```python
from build123d import *

# Parameters (mm, degrees)
BOSS_EXTRUDE1_DEPTH     = 18
CUT_EXTRUDE1_DEPTH      = 44.04814257
CUT_EXTRUDE1_DEPTH_BACK = 44.04814257
SKETCH5_R               = 1.5
CUT_EXTRUDE2_DEPTH      = 44.048142727
CUT_EXTRUDE3_START      = -18
CUT_EXTRUDE3_DEPTH      = 18
FILLET1_R               = 2
CUT_EXTRUDE5_REACH      = 44.569


# Read off the part's stored shape, not the designer's step: Cut-Extrude3
with BuildPart() as part:
    # Sketch2 → Boss-Extrude1 (new body)
    with BuildSketch(Plane(origin=(0, 0, 0), x_dir=(1, 0, 0), z_dir=(0, 1, 0))):
        with BuildLine():
            Line((5.149404736, 36.639918543), (4.036019928, 28.717773994))
            Line((4.036019928, 28.717773994), (-9.918584156, 27.251086003))
            Line((-9.918584156, 27.251086003), (-12.654745303, 34.768626969))
            ThreePointArc((-12.654745303, 34.768626969), (-3.867553141, 36.797310129), (5.149404736, 36.639918543))
        make_face()
    extrude(amount=BOSS_EXTRUDE1_DEPTH)

    # Sketch3 → Cut-Extrude1 (cut, two sides: drawn at the far end of the back side and taken through both)
    with BuildSketch(Plane(origin=(0, 0, 0), x_dir=(0, 0, -1), z_dir=(1, 0, 0)).offset(-CUT_EXTRUDE1_DEPTH_BACK)):
        with BuildLine():
            Line((38, 13.1), (41.639918543, 13.1))
            Line((41.639918543, 13.1), (41.639918543, 4.9))
            Line((41.639918543, 4.9), (38, 4.9))
            ThreePointArc((38, 4.9), (33.9, 9), (38, 13.1))
        make_face()
    extrude(amount=CUT_EXTRUDE1_DEPTH + CUT_EXTRUDE1_DEPTH_BACK, mode=Mode.SUBTRACT)

    # Sketch5 → Cut-Extrude2 (cut, through all)
    with BuildSketch(Plane.XY):
        with Locations(Location((0, 3.1, 0), (0, 0, 90))):
            Circle(SKETCH5_R)
        with Locations(Location((0, 14.9, 0), (0, 0, 90))):
            Circle(SKETCH5_R)
    extrude(amount=-CUT_EXTRUDE2_DEPTH, mode=Mode.SUBTRACT)

    # Cut-Extrude3 outline → Cut-Extrude3 (cut)
    with BuildSketch(Plane(origin=(0, 18, 0), x_dir=(1, 0, 0), z_dir=(0, 1, 0)).offset(CUT_EXTRUDE3_START)):
        with BuildLine():
            ThreePointArc((-12.483737701, 34.29877976), (-3.815290216, 36.300049044), (5.079818185, 36.144784509))
            Line((5.079818185, 36.144784509), (5.149404736, 36.639918543))
            ThreePointArc((5.149404736, 36.639918543), (-3.867553141, 36.797310129), (-12.654745303, 34.768626969))
            Line((-12.654745303, 34.768626969), (-12.483737701, 34.29877976))
        make_face()
    extrude(amount=CUT_EXTRUDE3_DEPTH, mode=Mode.SUBTRACT)

    # Fillet1
    fillet1_edges = [part.edges().sort_by_distance(p)[0] for p in [
        (4.557919056, 18, -32.431279251),
        (4.557919056, 0, -32.431279251),
        (-11.201159694, 0, -30.774933331),
        (-11.201159694, 18, -30.774933331),
    ]]
    fillet(fillet1_edges, radius=FILLET1_R)

    # Cut-Extrude5: up to this plane
    cut_extrude5_end = Plane(origin=(-10.179905315, 18, -29.737390741), z_dir=(-0.10452846326765396, 0, -0.9945218953682733))
    # Sketch7 → Cut-Extrude5 (cut, up to the surface)
    with BuildSketch(Plane.XY, mode=Mode.PRIVATE) as cut_extrude5_sk1:
        Polygon((3.233161507, 14.9), (1.616580754, 17.7), (-1.616580754, 17.7), (-3.233161507, 14.9), (-1.616580754, 12.1), (1.616580754, 12.1), align=None)
    cut_extrude5_tool1 = split(extrude(cut_extrude5_sk1.sketch, amount=-CUT_EXTRUDE5_REACH, mode=Mode.PRIVATE), bisect_by=cut_extrude5_end, keep=Keep.BOTH, mode=Mode.PRIVATE)
    add(cut_extrude5_tool1.solids().sort_by_distance((0, 14.9, 0))[0], mode=Mode.SUBTRACT)
    # Sketch7 → Cut-Extrude5 (cut, up to the surface)
    with BuildSketch(Plane.XY, mode=Mode.PRIVATE) as cut_extrude5_sk2:
        Polygon((-3.233161507, 3.1), (-1.616580754, 0.3), (1.616580754, 0.3), (3.233161507, 3.1), (1.616580754, 5.9), (-1.616580754, 5.9), align=None)
    cut_extrude5_tool2 = split(extrude(cut_extrude5_sk2.sketch, amount=-CUT_EXTRUDE5_REACH, mode=Mode.PRIVATE), bisect_by=cut_extrude5_end, keep=Keep.BOTH, mode=Mode.PRIVATE)
    add(cut_extrude5_tool2.solids().sort_by_distance((0, 3.1, 0))[0], mode=Mode.SUBTRACT)


solid = part.part
```
The model under review builds one solid part; all positions refer to its coordinate system, in mm. A direction names the side the tool comes from. Round coordinates to 2 decimals unless told otherwise and drop trailing zeros. Loops run counter-clockwise (first coordinate to the right, second up) from the corner with the lowest first, then second, coordinate; pieces in that order, holes last. Notation, with made-up numbers: (-6, 6) - (24, 6) arc R4 ccw to (24, 10) - close; hole circle Ø4 at (24, 74.5). An arc over 180 degrees is marked (long way). Use a Markdown table: item, result. Add a question column.
Q1. Machinability: for faces 4 (the face through (0, 5.9, -30)), 5 (the face through (-4, 0, -32)), which of the approach directions +Z, -Z, +X, -X, +Y, -Y give a long, thin tool a straight path to every point of the face, cutting with its end or side? Answer none if there is none.
Q2. Add section A-A (x = 1.25). State the section outline as (y, z) points.
Q3. The part is to be moulded in two halves that separate along X. For faces 1 (the face through (-2.436, 13.52, -29.277)), 2 (the face through (-3.939, 15.135, -36.287)), 3 (the face through (-3.8, 8.9, -33.9)), say which applies: pulls with the +X half, pulls with the -X half, needs draft (parallel to the pull), parting line crosses it, or undercut.
Q4. Add section D-D (y = 14.25). State the section outline as (x, z) points, plus the area to 3 significant figures.
Q5. Add section C-C (x = -6.5). State the section outline as (y, z) points.
Q6. Insertion check: pin 1 Ø2 at (y, z) = (10, -30.5) entering from +X; pin 2 Ø2 at (x, y) = (1, 9.5) entering from -Z; pin 3 Ø2 at (y, z) = (3, -31) entering from -X; pin 4 Ø3 at (x, z) = (-10.5, -32) entering from -Y. Each pin has a flat end and moves straight along its axis. Give the tip position at first contact, or say it passes through.
Q7. For probe 1 along Y at (x, z) = (-2.5, -30.5); probe 2 along Y at (x, z) = (-2.25, -28.25); probe 3 along X at (y, z) = (3.1, -33.9), list the stretches that pass through material, from the lowest coordinate up.
Q8. Add section B-B (y = 2.5). State the section outline as (x, z) points.
Worked answers:
| question | item | result |
|---|---|---|
| 1 | face 4 | +Z |
| 1 | face 5 | +Z, -Z, +X, -X, -Y |
| 2 | outline | (0, -36.48) - (2.27, -36.48) - (2.27, -30.94) - (0.3, -30.94) - (0.3, -28.42) - (0, -28.42) - close; (3.93, -36.48) - (5.19, -36.48) arc R4.1 cw to (12.81, -36.48) - (14.07, -36.48) - (14.07, -30.94) - (12.1, -30.94) - (12.1, -28.42) - (5.9, -28.42) - (5.9, -30.94) - (3.93, -30.94) - close; (15.73, -36.48) - (18, -36.48) - (18, -28.42) - (17.7, -28.42) - (17.7, -30.94) - (15.73, -30.94) - close |
| 3 | face 1 | undercut |
| 3 | face 2 | parting line crosses it |
| 3 | face 3 | needs draft |
| 4 | outline | (-12.48, -34.3) arc R36.5 ccw to (-1.35, -36.47) - (-1.35, -30.67) - (-2.86, -30.51) - (-2.86, -27.99) - (-9.92, -27.25) - close; (1.35, -36.47) arc R36.5 ccw to (5.08, -36.14) - (4.04, -28.72) - (2.86, -28.59) - (2.86, -31.11) - (1.35, -30.95) - close |
| 4 | area | 98.4 mm² |
| 5 | outline | (0, -35.92) - (5.47, -35.92) arc R4.1 cw to (12.53, -35.92) - (18, -35.92) - (18, -27.61) - (0, -27.61) - close |
| 6 | pin 1 | x = 4.43 |
| 6 | pin 2 | z = -34.18 |
| 6 | pin 3 | x = -11.65 |
| 6 | pin 4 | y = 0 |
| 7 | probe 1 | 0 to 1.83, 4.37 to 13.63, 16.17 to 18 |
| 7 | probe 2 | 0 to 1.4, 4.8 to 13.2, 16.6 to 18 |
| 7 | probe 3 | -12.34 to -1.5, 1.5 to 4.76 |
| 8 | outline | (-12.48, -34.3) arc R36.5 ccw to (-1.37, -36.47) - (-1.37, -30.66) - (-2.89, -30.5) - (-2.89, -27.99) - (-9.92, -27.25) - close; (1.37, -36.47) arc R36.5 ccw to (5.08, -36.14) - (4.04, -28.72) - (2.89, -28.6) - (2.89, -31.11) - (1.37, -30.95) - close |
